The listing builds one solid part. Answer for the finished solid, in the listing's coordinates (mm). Face numbers are marked on the shaded views. Coordinates: 2 decimals unless noted, no trailing zeros. Order: outer loops, then holes, each group sorted by start corner. A loop starts at its lowest first (then second) coordinate and runs counter-clockwise, first axis right, second up. Notation, with made-up numbers: M 13.5,-34.5 L 32.5,-34.5 A8 ccw 32.5,-20.5 Z; hole C -12,50.25 d8. An arc over 180 degrees is marked long. One line per item, written item: value. Start each with the question number.
Q1. Determine the mould class of the marked faces 1, 2 and 3 for opening direction X: pulls with the +X half, pulls with the -X half, needs draft (parallel to the pull), parting line crosses it, or undercut.
Q2. Straight lines are drawn through the part: line 1 along Z through (x, y) = (24, 58); line 2 along Y through (x, z) = (17.5, 47.5); line 3 along Y through (x, z) = (-4, 45). For each, find the intervals that lie inside material, in ascending order. Write a range as [from, to].
Q3. The part is cut by section D-D on z = 45.5. Give the vertices of the cut face in (x, y) (1 decimal), then the cut area to 3 significant figures.
Q4. Each of these flat-tipped pins is pushed along its axis until it touches: pin 1 Ø10 at (x, z) = (8.5, 76) entering from -Y; pin 2 Ø10 at (x, y) = (5, 79) entering from +Z; pin 3 Ø2 at (x, z) = (0, 80) entering from +Y. Where does it stop, or does it pass through?
Q5. The part is cut by section A-A on x = 14. Give the vertices of the cut face in (y, z), then the cut area to 3 significant figures.
Q6. The part is cut by section C-C on y = 68.5. Give the vertices of the cut face in (x, z).
Q7. The part is cut by section B-B on z = 5. Give the number of separate pieces and of enclosed holes in the cut face, then the cut area to 3 significant figures.
```python
from build123d import *

# Parameters (mm, degrees)
F1_DEPTH = 88.9
F3_W     = 62.738
F3_H     = 17.8308
F4_DEPTH = 63.5
F5_R     = 6.35
F6_DEPTH = 25.4


with BuildPart() as f1:
    # F0 (on Top) → F1 (new body)
    with BuildSketch(Plane.XY):
        with BuildLine():
            ThreePointArc((-18.647595, 22.647887), (0, 29.337), (18.647595, 22.647887))
            Line((18.647595, 22.647887), (31.4916, 34.48949))
            ThreePointArc((31.4916, 34.48949), (0.1226, 46.715736), (-31.2464, 34.48949))
            Line((-31.2464, 34.48949), (-18.647595, 22.647887))
        make_face()
    extrude(amount=F1_DEPTH)

    # F3 (on offset) → F4 (join)
    with BuildSketch(Plane.XZ.offset(-34.721038)):
        with Locations((0.1226, 8.9154)):
            Rectangle(F3_W, F3_H)
    extrude(amount=-F4_DEPTH)

    # F5 (on face) → F6 (cut)
    with BuildSketch(Plane.XY.offset(17.8308)):
        with Locations((18.7916, 85.521038)):
            Circle(F5_R)
        with Locations((-18.5464, 85.521038)):
            Circle(F5_R)
    extrude(amount=-F6_DEPTH, mode=Mode.SUBTRACT)


solid = f1.part
```
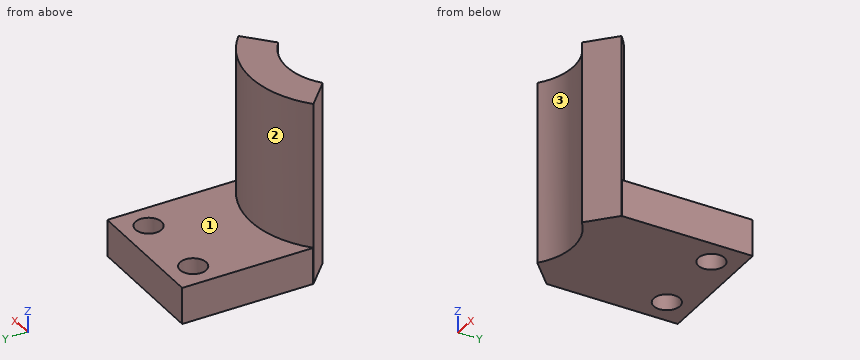
Output:
1. face 1: needs draft
1. face 2: parting line crosses it
1. face 3: undercut
2. line 1: z = [0, 17.83]
2. line 2: y = [23.55, 43.34]
2. line 3: y = [29.06, 46.53]
3. outline: M -31.2,34.5 L -18.6,22.6 A29.3 cw 18.6,22.6 L 31.5,34.5 A46.4 ccw Z
3. area: 948 mm^2
4. pin 1: stops at y = 26.05
4. pin 2: stops at z = 17.83
4. pin 3: stops at y = 46.72
5. outline: M 25.78,0 L 81.35,0 L 81.35,17.83 L 44.59,17.83 L 44.59,88.9 L 25.78,88.9 Z; M 89.69,0 L 98.22,0 L 98.22,17.83 L 89.69,17.83 Z
5. area: 2,480 mm^2
6. outline: M -31.25,0 L 31.49,0 L 31.49,17.83 L -31.25,17.83 Z
7. separate pieces: 1
7. enclosed holes: 2
7. area: 4,170 mm^2
